from build123d import *

# Parameters (mm, degrees)
SKETCH_1_R          = 55
EXTRUDE_1_DEPTH     = 1.5
SKETCH_2_W          = 41
SKETCH_2_H          = 20
CUT_EXTRUDE_1_DEPTH = 1.5
SKETCH_3_R          = 1.5
EXTRUDE_3_DEPTH     = 34
EXTRUDE_START       = 15.35
SKETCH_3_3_R        = 1.5
EXTRUDE_4_DEPTH     = 15.35


with BuildPart() as part:
    # Sketch 1 → Extrude 1 (new body)
    with BuildSketch(Plane(origin=(0, 0, 0), x_dir=(1, 0, 0), z_dir=(0, 1, 0))):
        with Locations(Location((0, 0, 0), (0, 0, 270))):
            Circle(SKETCH_1_R)
    extrude(amount=EXTRUDE_1_DEPTH)

    # Sketch 2 → Cut-Extrude 1 (cut)
    with BuildSketch(Plane(origin=(0, 1.5, 0), x_dir=(1, 0, 0), z_dir=(0, 1, 0))):
        with Locations((-10.5, 0)):
            Rectangle(SKETCH_2_W, SKETCH_2_H)
    extrude(amount=-CUT_EXTRUDE_1_DEPTH, mode=Mode.SUBTRACT)

    # Sketch 3 → Extrude 3 (add)
    # profile 1 of 4: a face of its own
    with BuildSketch(Plane(origin=(0, 1.5, 0), x_dir=(1, 0, 0), z_dir=(0, 1, 0))):
        Polygon((-2.5, 47.556624327), (0, 46.113248654), (2.5, 47.556624327), (2.5, 50.443375673), (0, 51.886751346), (-2.5, 50.443375673), align=None)
        with Locations(Location((0, 49, 0), (0, 0, 270))):
            Circle(SKETCH_3_R, mode=Mode.SUBTRACT)
    # profile 2 of 4: a face of its own
    with BuildSketch(Plane(origin=(0, 1.5, 0), x_dir=(1, 0, 0), z_dir=(0, 1, 0))):
        Polygon((-46.113248654, 0), (-47.556624327, 2.5), (-50.443375673, 2.5), (-51.886751346, 0), (-50.443375673, -2.5), (-47.556624327, -2.5), align=None)
        with Locations(Location((-49, 0, 0), (0, 0, 270))):
            Circle(SKETCH_3_R, mode=Mode.SUBTRACT)
    # profile 3 of 4: a face of its own
    with BuildSketch(Plane(origin=(0, 1.5, 0), x_dir=(1, 0, 0), z_dir=(0, 1, 0))):
        Polygon((47.556624327, 2.5), (46.113248654, 0), (47.556624327, -2.5), (50.443375673, -2.5), (51.886751346, 0), (50.443375673, 2.5), align=None)
        with Locations(Location((49, 0, 0), (0, 0, 270))):
            Circle(SKETCH_3_R, mode=Mode.SUBTRACT)
    # profile 4 of 4: a face of its own
    with BuildSketch(Plane(origin=(0, 1.5, 0), x_dir=(1, 0, 0), z_dir=(0, 1, 0))):
        Polygon((2.5, -47.556624327), (0, -46.113248654), (-2.5, -47.556624327), (-2.5, -50.443375673), (0, -51.886751346), (2.5, -50.443375673), align=None)
        with Locations(Location((0, -49, 0), (0, 0, 270))):
            Circle(SKETCH_3_R, mode=Mode.SUBTRACT)
    extrude(amount=-EXTRUDE_3_DEPTH)

    # Sketch 3_3 → Extrude 4 (add)
    # profile 1 of 4: a face of its own
    with BuildSketch(Plane(origin=(0, 1.5, 0), x_dir=(1, 0, 0), z_dir=(0, 1, 0)).offset(EXTRUDE_START)):
        Polygon((-2.5, 47.556624327), (0, 46.113248654), (2.5, 47.556624327), (2.5, 50.443375673), (0, 51.886751346), (-2.5, 50.443375673), align=None)
        with Locations(Location((0, 49, 0), (0, 0, 270))):
            Circle(SKETCH_3_3_R, mode=Mode.SUBTRACT)
    # profile 2 of 4: a face of its own
    with BuildSketch(Plane(origin=(0, 1.5, 0), x_dir=(1, 0, 0), z_dir=(0, 1, 0)).offset(EXTRUDE_START)):
        Polygon((-46.113248654, 0), (-47.556624327, 2.5), (-50.443375673, 2.5), (-51.886751346, 0), (-50.443375673, -2.5), (-47.556624327, -2.5), align=None)
        with Locations(Location((-49, 0, 0), (0, 0, 270))):
            Circle(SKETCH_3_3_R, mode=Mode.SUBTRACT)
    # profile 3 of 4: a face of its own
    with BuildSketch(Plane(origin=(0, 1.5, 0), x_dir=(1, 0, 0), z_dir=(0, 1, 0)).offset(EXTRUDE_START)):
        Polygon((47.556624327, 2.5), (46.113248654, 0), (47.556624327, -2.5), (50.443375673, -2.5), (51.886751346, 0), (50.443375673, 2.5), align=None)
        with Locations(Location((49, 0, 0), (0, 0, 270))):
            Circle(SKETCH_3_3_R, mode=Mode.SUBTRACT)
    # profile 4 of 4: a face of its own
    with BuildSketch(Plane(origin=(0, 1.5, 0), x_dir=(1, 0, 0), z_dir=(0, 1, 0)).offset(EXTRUDE_START)):
        Polygon((2.5, -47.556624327), (0, -46.113248654), (-2.5, -47.556624327), (-2.5, -50.443375673), (0, -51.886751346), (2.5, -50.443375673), align=None)
        with Locations(Location((0, -49, 0), (0, 0, 270))):
            Circle(SKETCH_3_3_R, mode=Mode.SUBTRACT)
    extrude(amount=-EXTRUDE_4_DEPTH)


solid = part.part
Geometry: final body of the model. Coordinates: model frame, mm. A direction names the side the tool comes from. Coordinates: 2 decimals unless noted, no trailing zeros. Order: outer loops, then holes, each group sorted by start corner. A loop starts at its lowest first (then second) coordinate and runs counter-clockwise, first axis right, second up. Notation, with made-up numbers: M 6,6.25 L 16,6.25 A14 cw 16,16.25 Z; hole C 40.25,63.5 d3. An arc over 180 degrees is marked long. One line per question, with ' | ' between items. Start each with the question number.
Item 1: Pin query (flat end, axial travel): pin 1 Ø2.5 at (x, z) = (0, -49) entering from -Y; pin 2 Ø1.2 at (y, z) = (1, 0) entering from -X; pin 3 Ø1.6 at (x, y) = (-16.5, 0.5) entering from +Z. Return the tip coordinate at first contact, or that it passes through.
Item 2: Cut plane D-D, the plane z = 4.5. Return the cut outline in (x, y), then the cut area to 3 significant figures.
Item 3: Cut plane B-B, the plane z = 49. Return the cut outline in (x, y).
Item 4: Cut plane C-C, the plane x = -27. Return the cut outline in (y, z), then the cut area to 3 significant figures.
Item 5: Set-up query: faces 1 (the flat face through (0, 0, 49)), 2 (the flat face through (2.5, 9, 49)), 3 (the flat face through (-46.845, 9.282, 1.267)). Return all of +Z, -Z, +X, -X, +Y, -Y with unobstructed straight access to the full face (end or side cutting, diameter ignored); none if empty.
Item 6: Cut plane A-A, the plane y = -2. Return the cut outline in (x, z), then the cut area to 3 significant figures.
Item 7: Ray query, probe 1 along X at (y, z) = (-22.5, 0); probe 2 along X at (y, z) = (12.75, -49); probe 3 along Y at (x, z) = (29, 19). Return the intervals inside material, ascending. Write a range as [from, to].
Item 8: Draft query along Z for faces 4 (the flat face through (-49, 9, 2.5)), 5 (the flat face through (-2.5, -16, -49)), 6 (the flat face through (-1.267, -16.022, -46.845)), 7 (the flat face through (-51.155, 9.282, -1.267)). Return one class per face: released by +Z, released by -Z, zero draft, split by the parting line, or undercut.
A:
1) pin 1: stops at y = 0 | pin 2: stops at x = -55 | pin 3: stops at z = 52.71
2) outline: M -54.82,0 L -31,0 L -31,1.5 L -54.82,1.5 Z; M 10,0 L 54.82,0 L 54.82,1.5 L 10,1.5 Z | area: 103 mm2
3) outline: M -24.98,0 L -2.5,0 L -2.5,-32.5 L -1.5,-32.5 L -1.5,0 L 1.5,0 L 1.5,-32.5 L 2.5,-32.5 L 2.5,0 L 24.98,0 L 24.98,1.5 L 2.5,1.5 L 2.5,16.85 L 1.5,16.85 L 1.5,1.5 L -1.5,1.5 L -1.5,16.85 L -2.5,16.85 L -2.5,1.5 L -24.98,1.5 Z
4) outline: M 0,-47.92 L 1.5,-47.92 L 1.5,-10 L 0,-10 Z; M 0,10 L 1.5,10 L 1.5,47.92 L 0,47.92 Z | area: 114 mm2
5) face 1: -Y | face 2: +Z, -Z, +X, +Y | face 3: +Z, +Y
6) outline: M -51.89,0 L -50.44,-2.5 L -47.56,-2.5 L -46.11,0 L -47.56,2.5 L -50.44,2.5 Z; M -2.5,-50.44 L 0,-51.89 L 2.5,-50.44 L 2.5,-47.56 L 0,-46.11 L -2.5,-47.56 Z; M -2.5,47.56 L 0,46.11 L 2.5,47.56 L 2.5,50.44 L 0,51.89 L -2.5,50.44 Z; M 46.11,0 L 47.56,-2.5 L 50.44,-2.5 L 51.89,0 L 50.44,2.5 L 47.56,2.5 Z; hole C -49,0 d3; hole C 0,-49 d3; hole C 0,49 d3; hole C 49,0 d3 | area: 58.3 mm2
7) probe 1: x = [-51.89, -50.5], [-47.5, -46.11], [46.11, 47.5], [50.5, 51.89] | probe 2: x = [-2.5, -1.5], [1.5, 2.5] | probe 3: y = [0, 1.5]
8) face 4: released by +Z | face 5: zero draft | face 6: undercut | face 7: released by -Z
